```python
from build123d import *

# Parameters (mm, degrees)
SKETCH_1_R               = 11.5
EXTRUDE_1_DEPTH          = 10
CHAMFER_1_SIZE           = 2
CHAMFER_2_SIZE           = 2
SKETCH_2_R               = 8.5
EXTRUDE_2_DEPTH          = 10
SKETCH_3_R               = 4.1
EXTRUDE_3_DEPTH          = 2
SKETCH_4_R               = 5
EXTRUDE_4_DEPTH          = 13
CHAMFER_3_SIZE           = 1
CUT_EXTRUDE_1_DEPTH      = 39.594040991
CUT_EXTRUDE_1_DEPTH_BACK = 39.594040991
SKETCH_5_R               = 2
CUT_EXTRUDE_2_DEPTH      = 39.594040991
CUT_EXTRUDE_2_DEPTH_BACK = 23
SKETCH_6_R               = 2


with BuildPart() as part:
    # Sketch 1 → Extrude 1 (new body)
    with BuildSketch(Plane(origin=(0, 0, 0), x_dir=(0, 0, -1), z_dir=(1, 0, 0))):
        Circle(SKETCH_1_R)
    extrude(amount=EXTRUDE_1_DEPTH)

    # Chamfer 1
    chamfer_1_edges = [part.edges().sort_by_distance(p)[0] for p in [
        (0, 0, 11.5),
    ]]
    chamfer(chamfer_1_edges, length=CHAMFER_1_SIZE)

    # Chamfer 2
    chamfer_2_edges = [part.edges().sort_by_distance(p)[0] for p in [
        (10, 0, 11.5),
    ]]
    chamfer(chamfer_2_edges, length=CHAMFER_2_SIZE)

    # Sketch 2 → Extrude 2 (add)
    with BuildSketch(Plane(origin=(10, 0, 0), x_dir=(0, 0, -1), z_dir=(1, 0, 0))):
        Circle(SKETCH_2_R)
    extrude(amount=EXTRUDE_2_DEPTH)

    # Sketch 3 → Extrude 3 (add)
    with BuildSketch(Plane(origin=(20, 0, 0), x_dir=(0, 0, -1), z_dir=(1, 0, 0))):
        Circle(SKETCH_3_R)
    extrude(amount=EXTRUDE_3_DEPTH)

    # Sketch 4 → Extrude 4 (add)
    with BuildSketch(Plane(origin=(22, 0, 0), x_dir=(0, 0, -1), z_dir=(1, 0, 0))):
        with Locations(Location((0, 0, 0), (0, 0, 180))):
            Circle(SKETCH_4_R)
    extrude(amount=EXTRUDE_4_DEPTH)

    # Chamfer 3
    chamfer_3_edges = [part.edges().sort_by_distance(p)[0] for p in [
        (35, 0, -5),
    ]]
    chamfer(chamfer_3_edges, length=CHAMFER_3_SIZE)

    # Sketch 5 → Cut-Extrude 1 (cut, two sides: drawn at the far end of the back side and taken through both)
    with BuildSketch(Plane.XY.offset(-CUT_EXTRUDE_1_DEPTH_BACK)):
        with Locations((15, 0)):
            Circle(SKETCH_5_R)
    extrude(amount=CUT_EXTRUDE_1_DEPTH + CUT_EXTRUDE_1_DEPTH_BACK, mode=Mode.SUBTRACT)

    # Sketch 6 → Cut-Extrude 2 (cut, two sides: drawn at the far end of the back side and taken through both)
    with BuildSketch(Plane(origin=(35, 0, 0), x_dir=(0, 0, -1), z_dir=(1, 0, 0)).offset(-CUT_EXTRUDE_2_DEPTH_BACK)):
        Circle(SKETCH_6_R)
    extrude(amount=CUT_EXTRUDE_2_DEPTH + CUT_EXTRUDE_2_DEPTH_BACK, mode=Mode.SUBTRACT)


solid = part.part
```
Could you check a few things on this model? Use its own coordinates, in mm. A direction names the side the tool comes from. Coordinates: 2 decimals unless noted, no trailing zeros. Write each loop counter-clockwise with the first axis right and the second up, starting at its lowest first coordinate (ties: lowest second). Pieces come first, ordered by that corner, then holes. Notation, with made-up numbers: (21.5, 28.5) -> (41.5, 28.5) arc R20 cw to (41.5, 58.5) -> close; hole circle Ø5 at (-13, 5). An arc over 180 degrees is marked (long way). Return JSON: item names as keys, results as strings.
(1) I'm going to push flat-ended pins straight in: pin 1 (10 mm diameter, centred on x = 13.5, y = 7, fed in from -Z); pin 2 (12 mm diameter, centred on x = 19, y = 4.5, fed in from -Z); pin 3 (3 mm diameter, centred on x = 6.5, y = 4.5, fed in from -Z). Where does each tip first touch, or does it pass through?
Numbers:
{"pin 1": "stops at z = -9.33", "pin 2": "stops at z = -8.5", "pin 3": "stops at z = -11.1"}
(2) Imagine slicing it at C-C, the plane x = 16.5. Please give me the cut outline in (y, z), then the cut area to 3 significant figures.
Numbers:
{"outline": "(-1.32, -8.4) -> (-1.32, -1.5) arc R2 cw to (-1.32, 1.5) -> (-1.32, 8.4) arc R8.5 ccw to start; (1.32, -8.4) arc R8.5 ccw to (1.32, 8.4) -> (1.32, 1.5) arc R2 cw to (1.32, -1.5) -> close", "area": "179 mm2"}
(3) I need wall thicknesses on L1, parallel to Y at x = 14.45, z = 0; L2, parallel to Y at x = 30, z = 0; L3, parallel to X at y = -0.5, z = -4.75. Which ranges of each line are inside material? Lowest first, please.
Numbers:
{"L1": "y = -8.5 to -2, 2 to 8.5", "L2": "y = -5 to -2, 2 to 5", "L3": "x = 0 to 13.06, 16.94 to 20, 22 to 34.22"}
(4) Imagine slicing it at A-A, the plane y = 0. Count the separate pieces of the cut face and the enclosed holes in it, then the cut area to 3 significant figures.
Numbers:
{"separate pieces": "3", "enclosed holes": "0", "area": "393 mm2"}
(5) We'd pull the mould along Z, two halves only. Please class faces 4 (the cylindrical face through (14.93, 2.55, -8.11)), 5 (the flat face through (0, 0, 0)), 6 (the cylindrical face through (13, 2, 0)): +Z half, -Z half, draft (parallel to the pull), parting line (faces both ways), or undercut.
Numbers:
{"face 4": "parting line", "face 5": "draft", "face 6": "undercut"}
(6) Imagine slicing it at B-B, the plane x = 32. Please give me the cut outline in (y, z).
Numbers:
{"outline": "circle Ø10 at (0, 0); hole circle Ø4 at (0, 0)"}
(7) Which directions (+Z, -Z, +X, -X, +Y, -Y) give clear straight access to the entire face, cutting with the end or side of a thin tool? Please do faces 1 (the cylindrical face through (5, 11.4, 1.5)), 2 (the cylindrical face through (20.986, 4.065, 0.534)), 3 (the cylindrical face through (28, 0, -5)).
Numbers:
{"face 1": "+X, -X", "face 2": "none", "face 3": "+X"}
